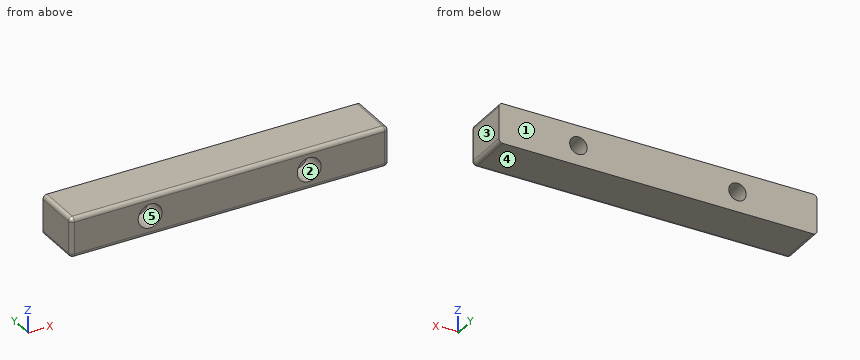
from build123d import *

# Parameters (mm, degrees)
F0_W     = 80
F0_H     = 12
F1_DEPTH = 10
F2_R     = 2.2
F3_DEPTH = 12.001
F2_R_2   = 3
F4_DEPTH = 6
F5_R     = 1


with BuildPart() as f1:
    # F0 (on Top) → F1 (new body)
    with BuildSketch(Plane.XY):
        Rectangle(F0_W, F0_H)
    extrude(amount=F1_DEPTH)

    # F2 (on face) → F3 (cut, through all)
    with BuildSketch(Plane.XZ.offset(6)):
        with Locations((-20, 5)):
            Circle(F2_R)
        with Locations((20, 5)):
            Circle(F2_R)
    extrude(amount=-F3_DEPTH, mode=Mode.SUBTRACT)

    # F2 (on face) → F4 (cut)
    with BuildSketch(Plane.XZ.offset(6)):
        with Locations((-20, 5)):
            Circle(F2_R_2)
        with Locations((-20, 5)):
            Circle(F2_R, mode=Mode.SUBTRACT)
        with Locations((20, 5)):
            Circle(F2_R_2)
        with Locations((20, 5)):
            Circle(F2_R, mode=Mode.SUBTRACT)
    extrude(amount=-F4_DEPTH, mode=Mode.SUBTRACT)

    # F5
    f5_edges = [f1.edges().sort_by_distance(p)[0] for p in [
        (0, -6, 10),
        (-40, 0, 10),
        (40, 0, 10),
        (-40, 0, 0),
        (0, -6, 0),
        (40, -6, 5),
        (-40, -6, 5),
        (40, 0, 0),
    ]]
    fillet(f5_edges, radius=F5_R)


solid = f1.part
Verification items for the finished model (mm, model axes). Face numbers are marked on the shaded views. A direction names the side the tool comes from. Give positions to 0.01 mm unless a question says otherwise; leave off trailing zeros. Order: outer loops, then holes, each group sorted by start corner. A loop starts at its lowest first (then second) coordinate and runs counter-clockwise, first axis right, second up. Notation, with made-up numbers: M 7,-22 L 41,-22 A18 cw 41,5 Z; hole C 3.25,88 d10. An arc over 180 degrees is marked long. Answer as a JSON object with one key per item and string values. Group by question number.
1) Access from +Z, -Z, +X, -X, +Y, -Y to the whole of each face (thin tool, end or side, straight path). Record for the marked faces 1 and 2.
2) Cross-section at D-D (y = -2.25). Enter the section's corners in (x, z), then the cut area to 3 significant figures.
3) Cross-section at A-A (z = 5). Enter the section's corners in (x, y), then the cut area to 3 significant figures.
4) Cross-section at C-C (y = 0.75). Enter the section's corners in (x, z).
5) Mould release check, pull along Z, two halves, no side actions. Record for the marked faces 3, 4 and 5: released by +Z, released by -Z, zero draft, split by the parting line, or undercut.
6) Cross-section at B-B (x = 20). Enter the section's corners in (y, z).
7) Scan lines: line 1 along Z through (x, y) = (20, 2.75); line 2 along X through (y, z) = (-5, 3.25); line 3 along X through (y, z) = (-3.5, 4.5). Record each from-to range of solid material in increasing order. Write a range as [from, to].
Result sheet:
{
 "1": {"face 1": "+Z, -Z, +X, -X, +Y", "face 2": "-Y"},
 "2": {"outline": "M -40,1 A1 ccw -39,0 L 39,0 A1 ccw 40,1 L 40,9 A1 ccw 39,10 L -39,10 A1 ccw -40,9 Z; hole C -20,5 d6; hole C 20,5 d6", "area": "743 mm2"},
 "3": {"outline": "M -40,-5 A1 ccw -39,-6 L -23,-6 L -23,0 L -22.2,0 L -22.2,6 L -40,6 Z; M -17.8,0 L -17,0 L -17,-6 L 17,-6 L 17,0 L 17.8,0 L 17.8,6 L -17.8,6 Z; M 22.2,0 L 23,0 L 23,-6 L 39,-6 A1 ccw 40,-5 L 40,6 L 22.2,6 Z", "area": "835 mm2"},
 "4": {"outline": "M -40,1 A1 ccw -39,0 L 39,0 A1 ccw 40,1 L 40,9 A1 ccw 39,10 L -39,10 A1 ccw -40,9 Z; hole C -20,5 d4.4; hole C 20,5 d4.4"},
 "5": {"face 3": "zero draft", "face 4": "released by -Z", "face 5": "undercut"},
 "6": {"outline": "M -6,1 A1 ccw -5,0 L 6,0 L 6,2.8 L 0,2.8 L 0,2 L -6,2 Z; M -6,8 L 0,8 L 0,7.2 L 6,7.2 L 6,10 L -5,10 A1 ccw -6,9 Z"},
 "7": {"line 1": "z = [0, 2.8], [7.2, 10]", "line 2": "x = [-40, -22.44], [-17.56, 17.56], [22.44, 40]", "line 3": "x = [-40, -22.96], [-17.04, 17.04], [22.96, 40]"}
}
